```python
from build123d import *

# Parameters (mm, degrees)
BOSS_EXTRUDE1_DEPTH     = 3.175
CUT_EXTRUDE1_DEPTH      = 135.971128857
CUT_EXTRUDE1_DEPTH_BACK = 135.971128857
SKETCH3_R               = 3.2
SKETCH6_R               = 1
SKETCH6_W               = 20
SKETCH6_H               = 3.175
CUT_EXTRUDE4_DEPTH      = 135.971128857
CUT_EXTRUDE5_DEPTH      = 135.971128857
CUT_EXTRUDE5_DEPTH_BACK = 135.971128857
SKETCH7_R               = 1
SKETCH7_W               = 4.8
SKETCH7_H               = 15
FILLET2_R               = 5
FILLET3_R               = 5
CUT_EXTRUDE6_DEPTH      = 135.971128857
CUT_EXTRUDE6_DEPTH_BACK = 135.971128857


with BuildPart() as part:
    # Sketch1 → Boss-Extrude1 (new body)
    with BuildSketch(Plane.XY):
        with BuildLine():
            Line((-111.101926123, 21.231014185), (-82, 20))
            Line((-82, 20), (25, 20))
            Line((25, 20), (25, -20))
            Line((25, -20), (-82, -20))
            Line((-82, -20), (-111.101926123, -21.231014185))
            ThreePointArc((-111.101926123, -21.231014185), (-133.25, 0), (-111.101926123, 21.231014185))
        make_face()
    extrude(amount=-BOSS_EXTRUDE1_DEPTH)

    # Sketch3 → Cut-Extrude1 (cut, two sides: drawn at the far end of the back side and taken through both)
    with BuildSketch(Plane.XY.offset(-CUT_EXTRUDE1_DEPTH_BACK)):
        with Locations((-110.75, 10)):
            Circle(SKETCH3_R)
    extrude(amount=CUT_EXTRUDE1_DEPTH + CUT_EXTRUDE1_DEPTH_BACK, mode=Mode.SUBTRACT)

    # Sketch6 → Cut-Extrude4 (cut, symmetric)
    with BuildSketch(Plane.XY):
        with Locations((9.5, 15.4125)):
            Circle(SKETCH6_R)
        with Locations((-27.5, 15.4125)):
            Circle(SKETCH6_R)
        with Locations((-9, 15.4125)):
            Rectangle(SKETCH6_W, SKETCH6_H)
    cut_extrude4 = extrude(amount=CUT_EXTRUDE4_DEPTH, both=True, mode=Mode.SUBTRACT)

    # Mirror1: Cut-Extrude4 across plane
    add(cut_extrude4.mirror(Plane.ZX), mode=Mode.SUBTRACT)

    # Sketch7 → Cut-Extrude5 (cut, two sides: drawn at the far end of the back side and taken through both)
    with BuildSketch(Plane.XY.offset(-CUT_EXTRUDE5_DEPTH_BACK)):
        with Locations((21.7875, 13)):
            Circle(SKETCH7_R)
        with Locations((21.7875, -13)):
            Circle(SKETCH7_R)
        with Locations((22.6, 0)):
            Rectangle(SKETCH7_W, SKETCH7_H)
    extrude(amount=CUT_EXTRUDE5_DEPTH + CUT_EXTRUDE5_DEPTH_BACK, mode=Mode.SUBTRACT)

    # Fillet2
    fillet2_edges = [part.edges().sort_by_distance(p)[0] for p in [
        (25, 20, -1.5875),
    ]]
    fillet(fillet2_edges, radius=FILLET2_R)

    # Fillet3
    fillet3_edges = [part.edges().sort_by_distance(p)[0] for p in [
        (25, -20, -1.5875),
    ]]
    fillet(fillet3_edges, radius=FILLET3_R)

    # Sketch8 → Cut-Extrude6 (cut, two sides: drawn at the far end of the back side and taken through both)
    with BuildSketch(Plane.XY.offset(-CUT_EXTRUDE6_DEPTH_BACK)):
        with BuildLine():
            Line((-107.55, -21.080767379), (-107.55, -1.160340262))
            ThreePointArc((-107.55, -1.160340262), (-110.75, 2.039659738), (-113.95, -1.160340262))
            Line((-113.95, -1.160340262), (-113.95, -21.160340262))
            ThreePointArc((-113.95, -21.160340262), (-112.527148786, -21.243460503), (-111.101926123, -21.231014185))
            Line((-111.101926123, -21.231014185), (-107.55, -21.080767379))
        make_face()
    extrude(amount=CUT_EXTRUDE6_DEPTH + CUT_EXTRUDE6_DEPTH_BACK, mode=Mode.SUBTRACT)


solid = part.part
```
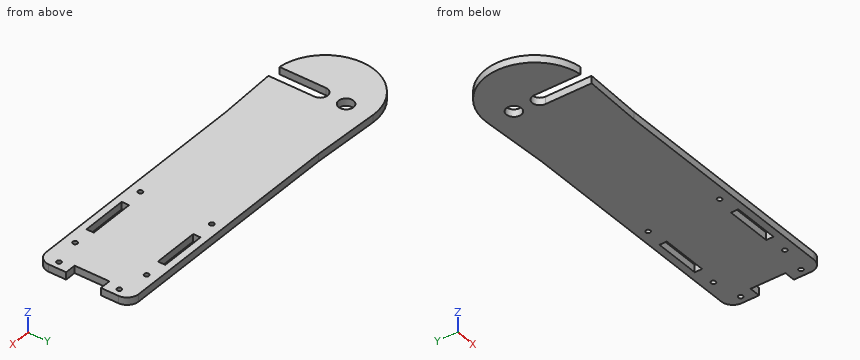
Geometry check sheet. Reference: the model listing, model coordinates, mm. Coordinates: 2 decimals unless noted, no trailing zeros. Order: outer loops, then holes, each group sorted by start corner. A loop starts at its lowest first (then second) coordinate and runs counter-clockwise, first axis right, second up.
Item 1: Scan lines: line 1 along Y through (x, z) = (9.5, -1.1); line 2 along X through (y, z) = (-13, -1.75); line 3 along Y through (x, z) = (1.5, -1.7). Record each from-to range of solid material in increasing order.
Item 2: Depth check by flat-ended pin: pin 1 (1.5 mm diameter, centred on y = -16, z = -2, fed in from +X); pin 2 (7.5 mm diameter, centred on x = -110.75, y = 10, fed in from -Z) (3 decimals); pin 3 (1.6 mm diameter, centred on x = 23.5, z = -1.5, fed in from -Y); pin 4 (1.6 mm diameter, centred on x = 21.79, y = 13, fed in from +Z). Enter the tip coordinate at first touch or a pass-through.
Item 3: Section check A-A (y = -5.5). Enter the section's corners in (x, z) (3 decimals).
Item 4: Section check B-B (z = -0.75). Count the separate pieces of the cut face and the enclosed holes in it, plus the area to 3 significant figures.
Item 5: Section check C-C (x = -61.5). Enter the section's corners in (y, z) (3 decimals).
Item 6: Section check D-D (x = -89). Enter the section's corners in (y, z) (3 decimals), plus the area to 3 significant figures.
Check sheet entries:
1. line 1: y = -20 to -16.41, -14.41 to 14.41, 16.41 to 20
1. line 2: x = -128.81 to -113.95, -107.55 to 20.79, 22.79 to 25
1. line 3: y = -20 to 20
2. pin 1: stops at x = 24.99
2. pin 2: stops at z = -3.175
2. pin 3: stops at y = -19.21
2. pin 4: passes through
3. outline: (-132.526, -3.175) - (-113.95, -3.175) - (-113.95, 0) - (-132.526, 0) - close; (-107.55, -3.175) - (20.2, -3.175) - (20.2, 0) - (-107.55, 0) - close
4. separate pieces: 1
4. enclosed holes: 9
4. area: 5,820 mm2
5. outline: (-20, -3.175) - (20, -3.175) - (20, 0) - (-20, 0) - close
6. outline: (-20.296, -3.175) - (20.296, -3.175) - (20.296, 0) - (-20.296, 0) - close
6. area: 129 mm2
